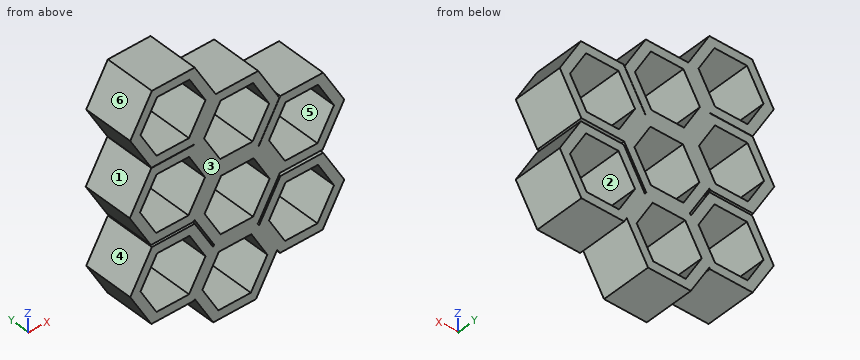
from build123d import *

# Parameters (mm, degrees)
F1_DEPTH = 25.4


with BuildPart() as f1:
    # F0 (on Front) → F1 (new body)
    with BuildSketch(Plane.XZ):
        Polygon((-37.5256026256, 45.1629495667), (-37.4485114416, 45.027359658), (-47.9911484283, 27.0428515349), (-37.8835519015, 9.2653571548), (-16.5829657817, 9.1244142096), (-16.054064132, 8.1941687175), (-15.6790532896, 8.1916873242), (-4.7170456877, 26.8915927664), (-15.4306350481, 45.7349225472), (-15.5873630008, 45.7359595938), (-15.927471531, 45.1557741399), (-37.4463405407, 45.2981614319), align=None)
        Polygon((-18.0099271589, 41.2211516747), (-9.9157319855, 26.8684398219), (-18.2984474766, 12.6823052521), (-34.7753581411, 12.8488825352), (-42.8695533144, 27.2015943881), (-34.4868378233, 41.3877289578), align=None, mode=Mode.SUBTRACT)
        Polygon((-47.9911484283, 27.0428515349), (-37.4485114416, 45.027359658), (-37.5256026256, 45.1629495667), (-48.0682396123, 27.1784414436), align=None)
        Polygon((-48.4105190435, 26.3274542158), (-47.9911484283, 27.0428515349), (-48.0682396123, 27.1784414436), (-37.5256026256, 45.1629495667), (-37.6030684933, 45.2991984785), (-48.1621008021, 63.8706894388), (-69.8376977643, 64.0141137774), (-80.7997053662, 45.3142083352), (-70.0861160058, 26.4708785543), align=None)
        Polygon((-50.7413929128, 59.3569185663), (-42.6471977395, 45.0042067135), (-51.0299132306, 30.8180721437), (-67.506823895, 30.9846494268), (-75.6010190684, 45.3373612797), (-67.2183035773, 59.5234958494), align=None, mode=Mode.SUBTRACT)
        Polygon((-16.5829657817, 9.1244142096), (-37.8835519015, 9.2653571548), (-37.3546502519, 8.3351116627), (-16.054064132, 8.1941687175), align=None)
        Polygon((-37.3546502519, 8.3351116627), (-37.8835519015, 9.2653571548), (-38.2585627439, 9.2678385482), (-38.5972650026, 8.6900520296), (-37.2000922861, 6.2326695996), (-47.8233976294, -11.889449324), (-38.5069809854, -28.2753966749), (-16.8313840231, -28.4188210135), (-6.0362439524, -10.003572102), (-15.430634824, 6.5195182768), (-15.2637672928, 6.8041748076), (-16.054064132, 8.1941687175), align=None)
        Polygon((-19.1622578925, 4.6106433371), (-11.0680627191, -9.7420685157), (-19.4507782102, -23.9282030855), (-35.9276888746, -23.7616258024), (-44.021884048, -9.4089139495), (-35.6391685569, 4.7772206202), align=None, mode=Mode.SUBTRACT)
        Polygon((-48.1621008021, 63.8706894388), (-37.6030684933, 45.2991984785), (-37.4463405407, 45.2981614319), (-37.1062320104, 45.8783468858), (-15.5873630008, 45.7359595938), (-4.9654639292, 63.8556795821), (-15.6790532896, 82.6990093629), (-37.2681492183, 82.8418613365), (-37.2000932002, 82.7221627042), (-48.1621008021, 64.022257262), (-48.2486018356, 64.022829627), align=None)
        Polygon((-18.2583454004, 78.1852384904), (-10.164150227, 63.8325266376), (-18.5468657181, 49.6463920679), (-35.0237763825, 49.8129693509), (-43.1179715559, 64.1656812038), (-34.7352560648, 78.3518157735), align=None, mode=Mode.SUBTRACT)
        Polygon((-37.1062320104, 45.8783468858), (-37.4463405407, 45.2981614319), (-15.927471531, 45.1557741399), (-15.5873630008, 45.7359595938), align=None)
        Polygon((-49.2205703458, -9.4320668941), (-38.5972650026, 8.6900520296), (-47.9136816466, 25.0759993804), (-69.5892786088, 25.219423719), (-80.5512862107, 6.5195182768), (-69.8376968503, -12.323811504), (-48.162099888, -12.4672358426), (-47.8233976294, -11.889449324), align=None)
        Polygon((-50.4929737574, 20.562228508), (-42.398778584, 6.2095166551), (-50.7814940751, -7.9766179146), (-67.2584047395, -7.8100406315), (-75.3525999129, 6.5426712213), (-66.9698844218, 20.7288057911), align=None, mode=Mode.SUBTRACT)
        Polygon((-37.2000922861, 6.2326695996), (-38.5972650026, 8.6900520296), (-49.2205703458, -9.4320668941), (-47.8233976294, -11.889449324), align=None)
        Polygon((-69.8376977643, 64.1656816006), (-48.2486018356, 64.022829627), (-48.3166578537, 64.1425282593), (-37.3546502519, 82.8424337015), (-37.2681492183, 82.8418613365), (-47.9136825606, 101.565492485), (-69.5892795229, 101.7089168236), (-80.5512871247, 83.0090113814), align=None)
        Polygon((-50.4929746714, 97.0517216126), (-42.398779498, 82.6990097597), (-50.7814949891, 68.51287519), (-67.2584056535, 68.6794524731), (-75.3526008269, 83.0321643259), (-66.9698853358, 97.2182988957), align=None, mode=Mode.SUBTRACT)
        Polygon((-48.3166578537, 64.1425282593), (-48.2486018356, 64.022829627), (-48.1621008021, 64.022257262), (-37.2000932002, 82.7221627042), (-37.2681492183, 82.8418613365), (-37.3546502519, 82.8424337015), align=None)
        Polygon((-5.8693764213, -9.7189155712), (-15.2637672928, 6.8041748076), (-15.430634824, 6.5195182768), (-6.0362439524, -10.003572102), align=None)
        Polygon((-4.4686272222, 25.219423719), (-15.2637672928, 6.8041748076), (-5.8693764213, -9.7189155712), (-6.0362439524, -10.003572102), (-4.7170454636, -12.323811504), (16.9585514987, -12.4672358426), (27.9205591005, 6.2326695996), (17.2069697401, 25.0759993804), align=None)
        Polygon((14.6276776293, 20.562228508), (22.7218728027, 6.2095166551), (14.3391573116, -7.9766179146), (-2.1377533528, -7.8100406315), (-10.2319485262, 6.5426712213), (-1.8492330351, 20.7288057911), align=None, mode=Mode.SUBTRACT)
        Polygon((-4.4686274462, 64.4348279895), (-15.4306350481, 45.7349225472), (-4.7170456877, 26.8915927664), (16.9585512746, 26.7481684278), (27.9205588764, 45.4480738701), (17.206969516, 64.2914036509), align=None)
        Polygon((14.6276774052, 59.7776327784), (22.7218725786, 45.4249209255), (14.3391570875, 31.2387863558), (-2.1377535769, 31.4053636389), (-10.2319487503, 45.7580754917), (-1.8492332592, 59.9442100615), align=None, mode=Mode.SUBTRACT)
    extrude(amount=F1_DEPTH)


solid = f1.part
Input: part model. Units: mm. Frame: model coordinates. Face numbers are marked on the shaded views. A direction names the side the tool comes from. Give positions to 0.01 mm unless a question says otherwise; leave off trailing zeros. Loops run counter-clockwise (first coordinate to the right, second up) from the corner with the lowest first, then second, coordinate; pieces in that order, holes last. Notation, with made-up numbers: (66.5, -21.5) -> (90.5, -21.5) arc R10 ccw to (90.5, -15.5) -> close; hole circle Ø4 at (53, 42.5). An arc over 180 degrees is marked (long way). Answer as a JSON object with one key per item and string values. Group by question number.
Item 1: Cut plane A-A, the plane z = 43. Return the cut outline in (x, y).
Item 2: Cut plane D-D, the plane x = -57. Return the cut outline in (y, z), and give its area (3 significant figures).
Item 3: Pin query (flat end, axial travel): P1, Ø1.5, axis at x = 2.5, y = -5, coming from the -Z side; P2, Ø5, axis at y = -18.5, z = 81.5, coming from the -X side; P3, Ø10, axis at x = -3.5, y = -15, coming from the +Z side. Return the tip coordinate at first contact, or that it passes through.
Item 4: Cut plane B-B, the plane x = 20.5. Return the cut outline in (y, z).
Item 5: Line query: probe 1 along Z at (x, y) = (-0.5, -15); probe 2 along Z at (x, y) = (-65, -6.25); probe 3 along X at (y, z) = (-17, 20). Output: solid intervals per line, ascending.
Item 6: Cut plane C-C, the plane z = -20. Return the cut outline in (x, y), and give its area (3 significant figures).
Item 7: Reachability of the marked faces 4, 5 and 6 from +Z, -Z, +X, -X, +Y, -Y: full face, straight path, thin tool, end or side. Return the list, or none.
Item 8: Pull-direction query (X, two-part tool) for the marked faces 1, 2 and 3; classes: released by +X, released by -X, zero draft, split by the parting line, or undercut.
Checks:
{
 "1": {"outline": "(-79.48, -25.4) -> (-74.28, -25.4) -> (-74.28, 0) -> (-79.48, 0) -> close; (-43.83, -25.4) -> (-8.68, -25.4) -> (-8.68, 0) -> (-43.83, 0) -> close; (21.29, -25.4) -> (26.49, -25.4) -> (26.49, 0) -> (21.29, 0) -> close"},
 "2": {"outline": "(-25.4, -12.41) -> (0, -12.41) -> (0, -7.91) -> (-25.4, -7.91) -> close; (-25.4, 20.63) -> (0, 20.63) -> (0, 25.14) -> (-25.4, 25.14) -> close; (-25.4, 26.38) -> (0, 26.38) -> (0, 30.88) -> (-25.4, 30.88) -> close; (-25.4, 59.42) -> (0, 59.42) -> (0, 63.93) -> (-25.4, 63.93) -> close; (-25.4, 64.08) -> (0, 64.08) -> (0, 68.58) -> (-25.4, 68.58) -> close; (-25.4, 97.12) -> (0, 97.12) -> (0, 101.63) -> (-25.4, 101.63) -> close", "area": "686 mm²"},
 "3": {"P1": "stops at z = -12.38", "P2": "stops at x = -80.55", "P3": "stops at z = 70.07"},
 "4": {"outline": "(-25.4, -6.43) -> (0, -6.43) -> (0, 2.45) -> (-25.4, 2.45) -> close; (-25.4, 10.15) -> (0, 10.15) -> (0, 19.28) -> (-25.4, 19.28) -> close; (-25.4, 32.79) -> (0, 32.79) -> (0, 41.66) -> (-25.4, 41.66) -> close; (-25.4, 49.36) -> (0, 49.36) -> (0, 58.5) -> (-25.4, 58.5) -> close"},
 "5": {"probe 1": "z = -12.35 to -7.83, 20.72 to 25.19, 26.86 to 31.39, 59.93 to 64.41", "probe 2": "z = -12.36 to -7.83, 20.71 to 25.19, 26.44 to 30.96, 59.5 to 63.98, 64.13 to 68.66, 97.2 to 101.68", "probe 3": "x = -72.65 to -67.4, -50.18 to -45.03, -43.99 to -38.81, -13.97 to -8.76, -7.53 to -2.28, 14.94 to 20.09"},
 "6": {"outline": "(-43.21, -25.4) -> (-38.05, -25.4) -> (-38.05, 0) -> (-43.21, 0) -> close; (-17.13, -25.4) -> (-11.9, -25.4) -> (-11.9, 0) -> (-17.13, 0) -> close", "area": "264 mm²"},
 "7": {"face 4": "-X, +Y, -Y", "face 5": "+Y, -Y", "face 6": "+Z, -X, +Y, -Y"},
 "8": {"face 1": "released by -X", "face 2": "undercut", "face 3": "zero draft"}
}
